Geometry: final body of the model. Coordinates: model frame, mm. A direction names the side the tool comes from. Give positions to 0.01 mm unless a question says otherwise; leave off trailing zeros. Write each loop counter-clockwise with the first axis right and the second up, starting at its lowest first coordinate (ties: lowest second). Pieces come first, ordered by that corner, then holes. Notation, with made-up numbers: (11.25, 67) -> (63.25, 67) arc R30 ccw to (63.25, 99) -> close; hole circle Ø7 at (13.25, 30.5). An arc over 180 degrees is marked (long way). Answer as a JSON object with one key per item and string values.
from build123d import *


with BuildPart() as f2:
    # F2: sweep along a path in F0
    with BuildLine(Plane.XY) as f2_path:
        Line((-51.5, -19), (51.5, -19))
        ThreePointArc((51.5, -19), (70.5, 0), (51.5, 19))
        Line((51.5, 19), (-51.5, 19))
        ThreePointArc((-51.5, 19), (-70.5, 0), (-51.5, -19))
    # F1 (on Right) → F2 (sweep)
    with BuildSketch(Plane.YZ):
        with BuildLine():
            Line((-7, -21.192692), (-7, -11.192692))
            ThreePointArc((-7, -11.192692), (-12.055502, -4.583723), (-19, 0))
            Line((-19, 0), (-19, -11.192692))
            Line((-19, -11.192692), (-19, -21.192692))
            Line((-19, -21.192692), (-7, -21.192692))
        make_face()
    sweep(path=f2_path.line)


solid = f2.part
Q1. Cut plane A-A (x = 5). Return the cut outline in (y, z), and give its area (3 significant figures).
Values:
{"outline": "(-19, -21.19) -> (-7, -21.19) -> (-7, -11.19) arc R25 ccw to (-19, 0) -> close; (7, -21.19) -> (19, -21.19) -> (19, 0) arc R25 ccw to (7, -11.19) -> close", "area": "405 mm²"}
Q2. First-contact query: P1, Ø6, axis at y = 10.5, z = -6.5, coming from the -X side; P2, Ø2, axis at x = 56, z = -15.5, coming from the -Y side; P3, Ø5, axis at x = -56.5, y = -3, coming from the +Z side; P4, Ø5, axis at x = 41.5, y = 2.5, coming from the -Z side. Flat tips, straight axial feed; report the tip coordinate or a pass-through.
Values:
{"P1": "x = -68.96", "P2": "y = -18.67", "P3": "z = -8.96", "P4": "through"}
Q3. Cut plane B-B (z = -12.5). Return the cut outline in (x, y).
Values:
{"outline": "(-51.5, -19) -> (51.5, -19) arc R19 ccw to (51.5, 19) -> (-51.5, 19) arc R19 ccw to start; hole (-51.5, -7) -> (51.5, -7) arc R7 ccw to (51.5, 7) -> (-51.5, 7) arc R7 ccw to start"}
Q4. Mould query, pull axis Y, two halves, no side actions, for faces 4 (the flat face through (-1, 19, -10)), 5 (the cylindrical face through (-58.5, 0.15, -16.12)), 6 (the flat face through (1, -19, -10)), 7 (the cylindrical face through (-0.721, 11.97, -4.664)). Classes: pulls with the +Y half, pulls with the -Y half, needs draft (parallel to the pull), parting line crosses it, or undercut.
Values:
{"face 4": "pulls with the +Y half", "face 5": "undercut", "face 6": "pulls with the -Y half", "face 7": "undercut"}
Q5. Set-up query: faces 1 (the cylindrical face through (0.721, -11.97, -4.664)), 2 (the flat face through (1, -7, -16)), 3 (the flat face through (1, -9, -21.193)). Return all of +Z, -Z, +X, -X, +Y, -Y with unobstructed straight access to the full face (end or side cutting, diameter ignored); none if empty.
Values:
{"face 1": "+Z", "face 2": "+Z, -Z", "face 3": "-Z, +X, -X, +Y, -Y"}
Q6. Material intervals for L1, parallel to Y at x = 1, z = -20; L2, parallel to X at y = 2, z = -11.25; L3, parallel to Y at x = -45, z = -3.25, sorted ascending. Write a range as from..to.
Values:
{"L1": "-19..-7, 7..19", "L2": "-70.39..-58.21, 58.21..70.39", "L3": "-19..-13.61, 13.61..19"}
Q7. Cut plane C-C (y = 0). Return the cut outline in (x, z).
Values:
{"outline": "(-70.5, -21.19) -> (-58.5, -21.19) -> (-58.5, -11.19) arc R25 ccw to (-70.5, 0) -> close; (58.5, -21.19) -> (70.5, -21.19) -> (70.5, 0) arc R25 ccw to (58.5, -11.19) -> close"}
Q8. Cut plane D-D (z = -5.5). Return the cut outline in (x, y), and give its area (3 significant figures).
Values:
{"outline": "(-51.5, -19) -> (51.5, -19) arc R19 ccw to (51.5, 19) -> (-51.5, 19) arc R19 ccw to start; hole (-51.5, -11.12) -> (51.5, -11.12) arc R11.12 ccw to (51.5, 11.12) -> (-51.5, 11.12) arc R11.12 ccw to start", "area": "2,370 mm²"}
